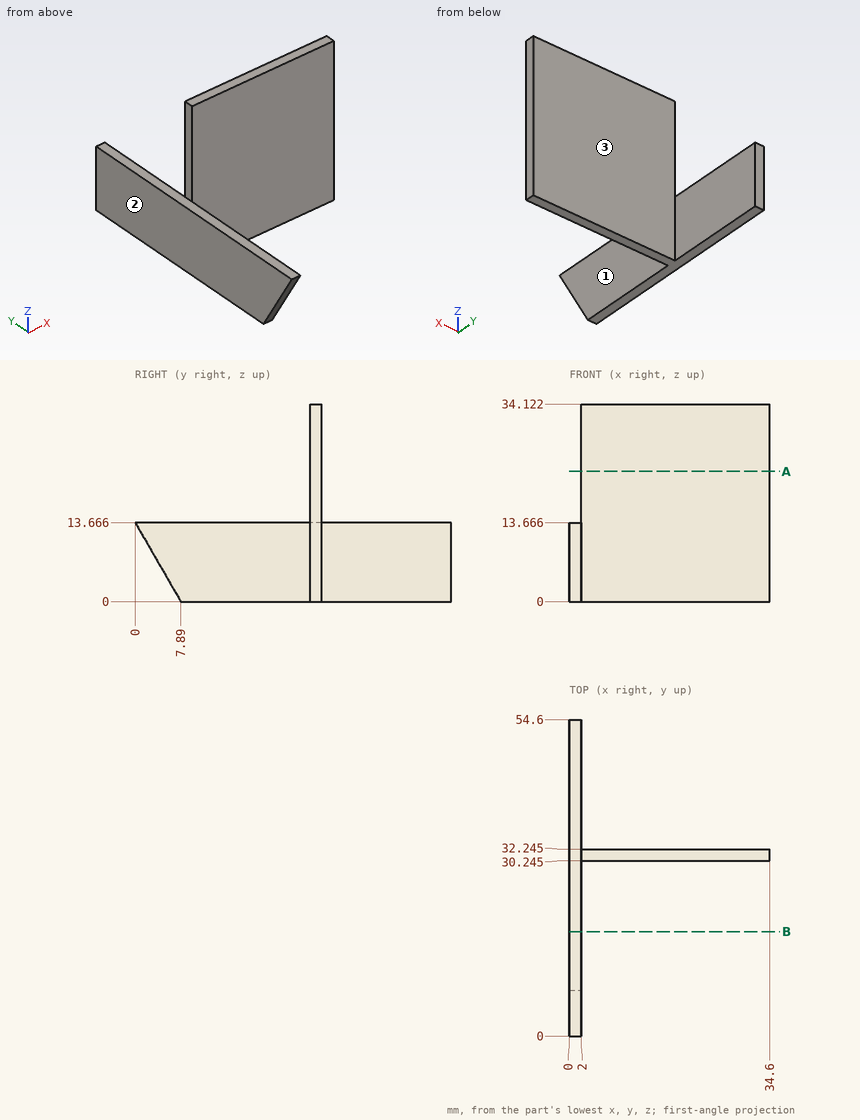
Drawing for the job (mm, zero at the part's lowest x, y, z). A direction names the side the tool comes from. Round coordinates to 2 decimals unless told otherwise and drop trailing zeros. Write each loop counter-clockwise with the first axis right and the second up, starting at its lowest first coordinate (ties: lowest second). Pieces come first, ordered by that corner, then holes. Notation, with made-up numbers: M 10.5,-3.5 L 55.5,-3.5 A22 cw 55.5,4.5 Z; hole C 39,3.5 d5. An arc over 180 degrees is marked long. Put each result on its own line as item: value.
Item 1: Tool access for the marked faces 1, 2 and 3: list every direction of +Z, -Z, +X, -X, +Y, -Y with a clear straight run to the whole face (end or side of a thin tool).
Responses:
face 1: +Z, -Z, +X, -Y
face 2: +Z, -Z, -X, +Y, -Y
face 3: +Z, -Z, +X, +Y
Item 2: Probe L1, parallel to Y at x = 23, z = 24 (3 decimals); L2, parallel to X at y = 3, z = 11; L3, parallel to X at y = 30.5, z = 19. List the from-to ranges inside material, lowest first. Write a range as from..to.
Responses:
L1: 30.245..32.245
L2: 0..2
L3: 2..34.6
Item 3: Cut at A-A (z = 22.5). List the corners of the cut face in (x, y) (3 decimals).
Responses:
outline: M 2,30.245 L 34.6,30.245 L 34.6,32.245 L 2,32.245 Z
Item 4: Flat gauge pins, fed straight in: P1, Ø8, axis at x = 23.5, z = 4, coming from the -Y side (3 decimals); P2, Ø2, axis at x = 25, z = 3.5, coming from the +Y side (3 decimals); P3, Ø1, axis at y = 31.5, z = 23, coming from the -X side. Where does each tip first touch, or does it go through?
Responses:
P1: y = 30.245
P2: y = 32.245
P3: x = 2
Item 5: Cut at B-B (y = 18). List the corners of the cut face in (x, z), and give its area (3 significant figures).
Responses:
outline: M 0,0 L 2,0 L 2,13.67 L 0,13.67 Z
area: 27.3 mm²
